Part model, mm, in its own coordinate system. A direction names the side the tool comes from. Give positions to 0.01 mm unless a question says otherwise; leave off trailing zeros. Loops run counter-clockwise (first coordinate to the right, second up) from the corner with the lowest first, then second, coordinate; pieces in that order, holes last. Notation, with made-up numbers: (57, 12.5) -> (100, 12.5) arc R20 cw to (100, 18.5) -> close; hole circle Ø8 at (24.5, 51.5). An arc over 180 degrees is marked (long way). One line per question, with ' | ' between items.
```python
from build123d import *

# Parameters (mm, degrees)
F2_R      = 4.1
F3_DEPTH  = 17
F4_R      = 2
F6_R      = 2
F7_DEPTH  = 12
F8_R      = 2
F9_SIZE   = 1
F10_R     = 1.5202998137
F11_DEPTH = 14


with BuildPart() as f1:
    # F0 (on Top) → F1 (revolve)
    with BuildSketch(Plane.XY):
        Polygon((13, -15), (7.821855842, 15), (0, 15), (0, -3.4), (8, -3.4), (8, -15), align=None)
    revolve(axis=Axis((0, 5.8, 0), (0, -1, 0)))

    # F2 (on face) → F3 (cut)
    with BuildSketch(Plane(origin=(0, 15, 0), x_dir=(-1, 0, 0), z_dir=(0, 1, 0))):
        Circle(F2_R)
    extrude(amount=-F3_DEPTH, mode=Mode.SUBTRACT)

    # F5: sweep along a path in F5_path
    with BuildLine(Plane(origin=(-4.1, -2, 0), x_dir=(0, 0, 1), z_dir=(0, -1, 0))) as f5_path:
        CenterArc((0, -4.1), 4.1, 0, 360)
    # F4 (on Right) → F5 (sweep, cut)
    with BuildSketch(Plane.YZ):
        with Locations((0, 3.7194299512)):
            Circle(F4_R)
    sweep(path=f5_path.line, mode=Mode.SUBTRACT)

    # F6 (on face) → F7 (cut)
    with BuildSketch(Plane(origin=(0, 15, 0), x_dir=(-1, 0, 0), z_dir=(0, 1, 0))):
        with Locations((-4.1, 0)):
            Circle(F6_R)
    extrude(amount=-F7_DEPTH, mode=Mode.SUBTRACT)

    # F8
    f8_edges = [f1.edges().sort_by_distance(p)[0] for p in [
        (-7.821856, 15, 0),
        (-13, -15, 0),
    ]]
    fillet(f8_edges, radius=F8_R)

    # F9
    f9_edges = [f1.edges().sort_by_distance(p)[0] for p in [
        (-8, -15, 0),
    ]]
    chamfer(f9_edges, length=F9_SIZE)

    # F10 (on face) → F11 (cut)
    with BuildSketch(Plane(origin=(0, 15, 0), x_dir=(-1, 0, 0), z_dir=(0, 1, 0))):
        with Locations((-3.9308541454, 0)):
            Circle(F10_R)
    extrude(amount=-F11_DEPTH, mode=Mode.SUBTRACT)


solid = f1.part
```
1) Tool access for faces 1 (the flat face through (-4.2, 15, -1.3)), 2 (the flat face through (0, -3.4, 0)), 3 (the cylindrical face through (-4.097, 8.573, -0.159)): list every direction of +Z, -Z, +X, -X, +Y, -Y with a clear straight run to the whole face (end or side of a thin tool).
Found:
face 1: +Z, -Z, +X, -X, +Y | face 2: -Y | face 3: +Y
2) Pin check, flat tips, straight feed: P1, Ø5, axis at x = -8.5, z = 2.5, coming from the +Y side; P2, Ø12, axis at y = 8.5, z = -3.5, coming from the -X side; P3, Ø3, axis at y = -7, z = -4, coming from the -X side. Stop position of each tip, or through.
Found:
P1: y = 14.99 | P2: x = -9.84 | P3: x = -11.44
3) Saw through at C-C (y = 12). Give the cut face in (x, z).
Found:
outline: circle Ø16.68 at (0, 0); hole (3.61, -1.94) arc R2 ccw (long way) to (3.61, 1.94) arc R4.1 ccw (long way) to start
4) Saw through at D-D (y = -0.5). Give the cut face in (x, z), and give its area (3 significant figures).
Found:
outline: circle Ø20.99 at (0, 0); hole circle Ø11.31 at (0, 0) | area: 246 mm2
5) Drill centre lines: line 1 (Y direction, x = 3.25, z = -0.75); line 2 (Y direction, x = -1.25, z = 6); line 3 (X direction, y = 1.8, z = 0). Where is each one in solid material? Low to high.
Found:
line 1: -3.4 to -2 | line 2: -3.4 to 15 | line 3: -10.1 to -4.59, 5.45 to 10.1
